Check sheet for the modelled part. Datum: model origin and axes. Units: mm. Face numbers are marked on the shaded views. A direction names the side the tool comes from. Round coordinates to 2 decimals unless told otherwise and drop trailing zeros. Loops run counter-clockwise (first coordinate to the right, second up) from the corner with the lowest first, then second, coordinate; pieces in that order, holes last. Notation, with made-up numbers: M 12.25,-38.5 L 42.25,-38.5 A36 ccw 42.25,-2.5 Z; hole C 88,62 d4. An arc over 180 degrees is marked long. Write item = value, one per line. Start each with the question number.
(1) Cross-section at D-D on y = 61.5. Record the boundary of the cut face in (x, z).
(2) Cross-section at A-A on z = -128.5. Record the boundary of the cut face in (x, y).
(3) Set-up check for the marked faces 5 and 6: record each of +Z, -Z, +X, -X, +Y, -Y from which the full face is reachable in a straight line by a thin tool's end or side.
(4) Scan lines: L1, parallel to Z at x = 13, y = 52; L2, parallel to Z at x = 133, y = 13.5; L3, parallel to X at y = 56, z = -90. Record each from-to range of solid material in increasing order. Write a range as from..to.
(5) Cross-section at C-C on x = 52. Record the boundary of the cut face in (y, z), plus the area to 3 significant figures.
(6) Cross-section at B-B on y = 76. Record the boundary of the cut face in (x, z), plus the area to 3 significant figures.
(7) Mould release check, pull along Z, two halves, no side actions. Record for the marked faces 1, 2, 3 and 4: pulls with the +Z half, pulls with the -Z half, needs draft (parallel to the pull), parting line crosses it, or undercut.
(8) Go/stop test with flat-tipped pins: P1, Ø4.5, axis at x = 19.5, y = 74, coming from the -Z side; P2, Ø12, axis at x = 121, y = 80, coming from the +Z side; P3, Ø2, axis at y = 81, z = 2.5, coming from the -X side. Record where each tip stops, or that it passes through.
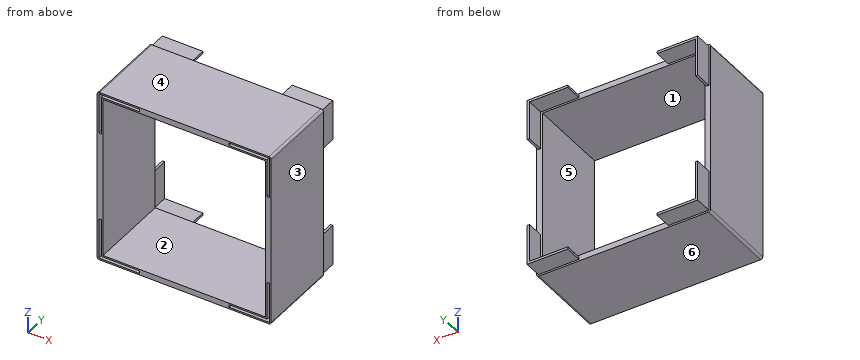
from build123d import *

# Parameters (mm, degrees)
SKETCH1_W           = 150
SKETCH1_H           = 150
SKETCH1_W_2         = 140
SKETCH1_H_2         = 140
BOSS_EXTRUDE1_DEPTH = 70
BOSS_EXTRUDE2_DEPTH = 15
CUT_EXTRUDE1_DEPTH  = 25
FILLET1_R           = 2


with BuildPart() as part:
    # Sketch1 → Boss-Extrude1 (new body)
    with BuildSketch(Plane(origin=(0, 0, 0), x_dir=(1, 0, 0), z_dir=(0, 1, 0))):
        with Locations((70, 70)):
            Rectangle(SKETCH1_W, SKETCH1_H)
        with Locations((70, 70)):
            Rectangle(SKETCH1_W_2, SKETCH1_H_2, mode=Mode.SUBTRACT)
    extrude(amount=BOSS_EXTRUDE1_DEPTH)

    # Sketch2 → Boss-Extrude2 (add)
    with BuildSketch(Plane(origin=(0, 70, 0), x_dir=(1, 0, 0), z_dir=(0, 1, 0))):
        Polygon((-3.5, 108.5), (-3.5, 143.5), (31.5, 143.5), (31.5, 141.5), (-1.5, 141.5), (-1.5, 108.5), align=None)
        Polygon((143.5, 108.5), (143.5, 143.5), (108.5, 143.5), (108.5, 141.5), (141.5, 141.5), (141.5, 108.5), align=None)
        Polygon((143.5, 31.5), (143.5, -3.5), (108.5, -3.5), (108.5, -1.5), (141.5, -1.5), (141.5, 31.5), align=None)
        Polygon((-3.5, 31.5), (-3.5, -3.5), (31.5, -3.5), (31.5, -1.5), (-1.5, -1.5), (-1.5, 31.5), align=None)
    extrude(amount=BOSS_EXTRUDE2_DEPTH)

    # Sketch3 → Cut-Extrude1 (cut)
    with BuildSketch(Plane.XZ):
        Polygon((-3.65, 3.65), (31.55, 3.65), (31.55, 1.35), (-1.35, 1.35), (-1.35, -31.55), (-3.65, -31.55), align=None)
        Polygon((143.65, -31.55), (143.65, 3.65), (108.45, 3.65), (108.45, 1.35), (141.35, 1.35), (141.35, -31.55), align=None)
        Polygon((143.65, -143.65), (108.45, -143.65), (108.45, -141.35), (141.35, -141.35), (141.35, -108.45), (143.65, -108.45), align=None)
        Polygon((-3.65, -108.45), (-3.65, -143.65), (31.55, -143.65), (31.55, -141.35), (-1.35, -141.35), (-1.35, -108.45), align=None)
    extrude(amount=-CUT_EXTRUDE1_DEPTH, mode=Mode.SUBTRACT)

    # Fillet1
    fillet1_edges = [part.edges().sort_by_distance(p)[0] for p in [
        (-5, 35, 5),
        (-5, 35, -145),
        (145, 35, -145),
        (145, 35, 5),
    ]]
    fillet(fillet1_edges, radius=FILLET1_R)


solid = part.part
Result:
q1.outline = M -5,-143 A2 ccw -3,-145 L 143,-145 A2 ccw 145,-143 L 145,3 A2 ccw 143,5 L -3,5 A2 ccw -5,3 Z; hole M 0,-140 L 140,-140 L 140,0 L 0,0 Z
q2.outline = M -5,0 L -3.65,0 L -3.65,25 L -1.35,25 L -1.35,0 L 0,0 L 0,70 L -1.5,70 L -1.5,85 L -3.5,85 L -3.5,70 L -5,70 Z; M 140,0 L 141.35,0 L 141.35,25 L 143.65,25 L 143.65,0 L 145,0 L 145,70 L 143.5,70 L 143.5,85 L 141.5,85 L 141.5,70 L 140,70 Z
q3.face_5 = +Y, -Y
q3.face_6 = -Z, +X, -X, +Y, -Y
q4.L1 = -145..-140, 0..5
q4.L2 = -145..-143.65, -141.35..-140, 0..1.35, 3.65..5
q4.L3 = -5..0, 140..145
q5.outline = M 0,-145 L 70,-145 L 70,-140 L 0,-140 Z; M 0,0 L 70,0 L 70,5 L 0,5 Z
q5.area = 700 mm^2
q6.outline = M -3.5,-143.5 L 31.5,-143.5 L 31.5,-141.5 L -1.5,-141.5 L -1.5,-108.5 L -3.5,-108.5 Z; M -3.5,-31.5 L -1.5,-31.5 L -1.5,1.5 L 31.5,1.5 L 31.5,3.5 L -3.5,3.5 Z; M 108.5,-143.5 L 143.5,-143.5 L 143.5,-108.5 L 141.5,-108.5 L 141.5,-141.5 L 108.5,-141.5 Z; M 108.5,1.5 L 141.5,1.5 L 141.5,-31.5 L 143.5,-31.5 L 143.5,3.5 L 108.5,3.5 Z
q6.area = 544 mm^2
q7.face_1 = undercut
q7.face_2 = undercut
q7.face_3 = needs draft
q7.face_4 = pulls with the +Z half
q8.P1 = -143.5
q8.P2 = 3.5
q8.P3 = -3.5
